Can you work these out from the model? Positions are in its coordinate system, mm. A direction names the side the tool comes from. Give positions to 0.01 mm unless a question says otherwise; leave off trailing zeros. Write each loop counter-clockwise with the first axis right and the second up, starting at its lowest first coordinate (ties: lowest second). Pieces come first, ordered by that corner, then holes.
1. Suppose I cut it at B-B (y = 8.75). Please give me the cut outline in (x, z), and give its area (3 significant figures).
2. Thinking about a two-plate mould opening in Z: for faces 1 (the cylindrical face through (0.07, 5.82, -1.5)), 2 (the flat face through (0, 1.2, 0)), 3 (the flat face through (-1.3, 0, 0)), which applies, pulls with the +Z half, pulls with the -Z half, needs draft (parallel to the pull), parting line crosses it, or undercut?
3. I'm going to push flat-ended pins straight in: pin 1 (1 mm diameter, centred on y = 1, z = 1.5, fed in from -X); pin 2 (3 mm diameter, centred on x = 0.5, y = 3, fed in from -Z); pin 3 (3 mm diameter, centred on y = 7.5, z = 2, fed in from -X). Where does each tip first touch, or does it pass through?
4. Suppose I cut it at A-A (z = 0). Please give me the cut outline in (x, y) (3 decimals).
5. If I drill on probe 1 along Y at (x, z) = (-1.2, 1.6); probe 2 along Y at (x, z) = (0.6, -0.35); probe 3 along X at (y, z) = (9, 0.25), over which ranges is the centre line in solid material (lowest first)?
6. On a 3-axis mill with a long thin cutter (end or side, diameter ignored), from which of +Z, -Z, +X, -X, +Y, -Y can I reach the whole of each face in a straight line? I mean faces 4 (the flat face through (-1, 1, 0)), 5 (the flat face through (0, 10, 0)). Say none if no direction works.
```python
from build123d import *

# Parameters (mm, degrees)
POCKET_DEPTH = 1.2


with BuildPart() as part:
    # Sketch → Revolution (revolve)
    with BuildSketch(Plane.YZ):
        Polygon((0, 0), (0, 3), (0.2, 3), (1.7, 1.5), (9.823908, 1.5), (10, 1.195), (10, 0), align=None)
    revolve(axis=Axis((0, 0, 0), (0, 1, 0)))

    # Sketch001 → Pocket (cut)
    with BuildSketch(Plane(origin=(0, 0, 0), x_dir=(0, 0, -1), z_dir=(0, -1, 0))):
        Polygon((0.57735, 1), (-0.57735, 1), (-1.154701, 0), (-0.57735, -1), (0.57735, -1), (1.154701, 0), align=None)
    extrude(amount=-POCKET_DEPTH, mode=Mode.SUBTRACT)


solid = part.part
```
Checks:
1. outline: circle Ø3 at (0, 0)
1. area: 7.07 mm2
2. face 1: parting line crosses it
2. face 2: undercut
2. face 3: needs draft
3. pin 1: stops at x = -2.32
3. pin 2: stops at z = -1.66
3. pin 3: stops at x = -1.41
4. outline: (-3, 0) - (-1, 0) - (-1, 1.2) - (1, 1.2) - (1, 0) - (3, 0) - (3, 0.2) - (1.5, 1.7) - (1.5, 9.824) - (1.195, 10) - (-1.195, 10) - (-1.5, 9.824) - (-1.5, 1.7) - (-3, 0.2) - close
5. probe 1: y = 0 to 1.2
5. probe 2: y = 1.2 to 10
5. probe 3: x = -1.48 to 1.48
6. face 4: -Y
6. face 5: +Z, -Z, +X, -X, +Y
